from build123d import *

# Parameters (mm, degrees)
F3_DEPTH = 15


with BuildPart() as f1:
    # F0 (on Right) → F1 (revolve)
    with BuildSketch(Plane.YZ):
        with BuildLine():
            Line((15, 12.25), (1.288e-07, 12.25))
            ThreePointArc((1.288e-07, 12.25), (-6.8897568365, 10.1288573262), (-11.3935288651, 4.5))
            Line((-11.3935288651, 4.5), (-10.3107953137, 4.5))
            ThreePointArc((-10.3107953137, 4.5), (-6.1618787719, 9.4124252985), (0, 11.25))
            Line((0, 11.25), (15, 11.25))
            Line((15, 11.25), (15, 12.25))
        make_face()
        with BuildLine():
            Line((-10.3107953137, 4.5), (-11.3935288651, 4.5))
            ThreePointArc((-11.3935288651, 4.5), (-11.7355401547, 3.5127762921), (-11.9921849552, 2.5))
            Line((-11.9921849552, 2.5), (-10.9687054842, 2.5))
            ThreePointArc((-10.9687054842, 2.5), (-10.6866406579, 3.5154247891), (-10.3107953137, 4.5))
        make_face()
        with BuildLine():
            ThreePointArc((-11.9921849552, 2.5), (-11.7355401547, 3.5127762921), (-11.3935288651, 4.5))
            Line((-11.3935288651, 4.5), (-12.25, 4.5))
            Line((-12.25, 4.5), (-12.25, 2.5))
            Line((-12.25, 2.5), (-11.9921849552, 2.5))
        make_face()
    revolve(axis=Axis((0, 1.375, 3.22e-08), (0, 1, -2.4e-09)))

    # F2 (on Right) → F3 (cut, symmetric)
    with BuildSketch(Plane.YZ):
        Polygon((-12.7222961238, 24.7129239332), (15, -12.25), (15, 24.7129239332), align=None)
    extrude(amount=F3_DEPTH, both=True, mode=Mode.SUBTRACT)


solid = f1.part
Build history of the part. All positions in model axes, mm. Give positions to 0.01 mm unless a question says otherwise; leave off trailing zeros. Loops run counter-clockwise (first coordinate to the right, second up) from the corner with the lowest first, then second, coordinate; pieces in that order, holes last. Notation, with made-up numbers: (20.25, 10.5) - (64.25, 10.5) arc R33 cw to (64.25, 40.5) - close; hole circle Ø11 at (62.25, 31). An arc over 180 degrees is marked (long way). Write item = value, one per line. Start each with the question number.
1) Probe probe 1 along Z at (x, y) = (0, 9); probe 2 along Z at (x, y) = (-1.75, -4); probe 3 along Z at (x, y) = (-3, 13.75). List the from-to ranges inside material, lowest first. Write a range as from..to.
2) Band-saw the part on D-D on y = -1.5. Give the cut face in (x, z).
3) Band-saw the part on C-C on z = -5. Give the cut face in (x, y), plus the area to 3 significant figures.
4) Band-saw the part on B-B on x = -6.5. Give the cut face in (y, z), plus the area to 3 significant figures.
5) Drop flat-ended pins along their axis: pin 1 Ø10 at (x, z) = (-7.5, -2) entering from +Y; pin 2 Ø6 at (y, z) = (-7.5, -1.5) entering from -X; pin 3 Ø2 at (x, z) = (-7, 8.5) entering from -Y. Give the stop position or say it passes through.
6) Pull direction X, two halves, no side cores. Call faces 1 (the cylindrical face through (0.367, 5.809, -11.244)), 2 (the cylindrical face through (2.11, -11.6, 1.34)), 3 (the flat face through (10.95, 3.24, 3.43)), 4 (the cylindrical face through (-4.39, -11.83, -0.98)): +X half, -X half, draft (parallel to the pull), parting line (faces both ways), or undercut.
7) Band-saw the part on A-A on z = -1.25. Give the cut face in (x, y), plus the area to 3 significant figures.
Final values:
q1.probe_1 = -12.25..-11.25
q1.probe_2 = -11.45..-10.37, 10.37..11.45
q1.probe_3 = -11.88..-10.84
q2.outline = (-7.26, 9.75) arc R12.16 ccw (long way) to (7.26, 9.75) - (5.41, 9.75) arc R11.15 cw (long way) to (-5.41, 9.75) - close
q3.outline = (-11.18, 0) arc R11.18 ccw to (11.18, 0) - (11.18, 9.56) - (10.08, 9.56) - (10.08, 0) arc R10.08 cw to (-10.08, 0) - (-10.08, 9.56) - (-11.18, 9.56) - close
q3.area = 58.1 mm²
q4.outline = (-1.85, 10.22) arc R10.38 ccw to (0, -10.38) - (13.6, -10.38) - (12.7, -9.18) - (0, -9.18) arc R9.18 cw to (-1.03, 9.12) - close
q4.area = 51.0 mm²
q5.pin_1 = 10.89
q5.pin_2 = -11.33
q5.pin_3 = -7.06
q6.face_1 = undercut
q6.face_2 = undercut
q6.face_3 = draft
q6.face_4 = parting line
q7.outline = (-12.19, 0) arc R12.19 ccw to (-4.32, -11.39) - (-4.32, -12.25) - (-2.17, -12.25) - (-2.17, -10.97) arc R11.18 cw to (-11.18, 0) - (-11.18, 6.75) - (-12.19, 6.75) - close; (2.17, -12.25) - (4.32, -12.25) - (4.32, -11.39) arc R12.19 ccw to (12.19, 0) - (12.19, 6.75) - (11.18, 6.75) - (11.18, 0) arc R11.18 cw to (2.17, -10.97) - close
q7.area = 48.4 mm²
